Input: part model. Units: mm. Frame: model coordinates. A direction names the side the tool comes from. Round coordinates to 2 decimals unless told otherwise and drop trailing zeros. Write each loop counter-clockwise with the first axis right and the second up, starting at its lowest first coordinate (ties: lowest second). Pieces come first, ordered by that corner, then holes. Notation, with made-up numbers: (89, 72) - (125, 72) arc R25 cw to (125, 101) - close; hole circle Ø5 at (2, 3.25). An arc over 180 degrees is marked (long way). Use one line per item in the form item = value.
```python
from build123d import *

# Parameters (mm, degrees)
BOSS_EXTRUDE1_DEPTH  = 6.35
M5_CLEARANCE_HOLE1_D = 5.5
CUT_EXTRUDE2_DEPTH   = 7.35
FILLET1_R            = 10
M3_CLEARANCE_HOLE1_D = 3.4
SKETCH10_R           = 11.5
CUT_EXTRUDE3_DEPTH   = 7.35
FILLET2_R            = 5


with BuildPart() as part:
    # Sketch1 → Boss-Extrude1 (new body)
    with BuildSketch(Plane(origin=(0, 0, 0), x_dir=(1, 0, 0), z_dir=(0, 1, 0))):
        with BuildLine():
            Line((25.4, -25.4), (-25.4, -25.4))
            Line((-25.4, -25.4), (-25.4, 25.4))
            Line((-25.4, 25.4), (-25.4, 43.35))
            Line((-25.4, 43.35), (1.2, 43.35))
            Line((1.2, 43.35), (1.2, 25.4))
            Line((1.2, 25.4), (25.4, 25.4))
            Line((25.4, 25.4), (89.621209859, 25.4))
            Line((89.621209859, 25.4), (89.621209859, -50.04))
            Line((89.621209859, -50.04), (51.541941751, -50.04))
            ThreePointArc((51.541941751, -50.04), (44.870841587, -48.474895705), (39.591870426, -44.10618968))
            Line((39.591870426, -44.10618968), (25.4, -25.4))
        make_face()
    extrude(amount=BOSS_EXTRUDE1_DEPTH)

    # M5 Clearance Hole1 (through all)
    with Locations(Plane(origin=(0, 6.35, 0), x_dir=(1, 0, 0), z_dir=(0, 1, 0))):
        with Locations((-12.7, 12.7), (12.7, 12.7), (12.7, -12.7), (-12.7, -12.7), (-11.5, 38.1)):
            Hole(M5_CLEARANCE_HOLE1_D / 2)

    # Sketch7 → Cut-Extrude2 (cut, through all)
    with BuildSketch(Plane(origin=(0, 6.35, 0), x_dir=(1, 0, 0), z_dir=(0, 1, 0))):
        with BuildLine():
            Line((53.051764766, -31.105892862), (50.215452987, -32.745892862))
            ThreePointArc((50.215452987, -32.745892862), (49.247834614, -36.366488764), (52.868430515, -37.334107138))
            Line((52.868430515, -37.334107138), (55.704742294, -35.694107138))
            ThreePointArc((55.704742294, -35.694107138), (56.672360668, -32.073511236), (53.051764766, -31.105892862))
        make_face()
        with BuildLine():
            Line((33.75, -19.08), (33.75, -20.72))
            ThreePointArc((33.75, -20.72), (36.4, -23.37), (39.05, -20.72))
            Line((39.05, -20.72), (39.05, -19.08))
            ThreePointArc((39.05, -19.08), (36.4, -16.43), (33.75, -19.08))
        make_face()
    extrude(amount=-CUT_EXTRUDE2_DEPTH, mode=Mode.SUBTRACT)

    # Fillet1
    fillet1_edges = [part.edges().sort_by_distance(p)[0] for p in [
        (-25.4, 3.175, -43.35),
        (1.2, 3.175, -43.35),
        (89.621209859, 3.175, -25.4),
        (89.621209859, 3.175, 50.04),
        (25.4, 3.175, 25.4),
        (-25.4, 3.175, 25.4),
    ]]
    fillet(fillet1_edges, radius=FILLET1_R)

    # M3 Clearance Hole1 (through all)
    with Locations(Plane(origin=(0, 6.35, 0), x_dir=(1, 0, 0), z_dir=(0, 1, 0))):
        with Locations((50.121209859, 9.14), (81.121209859, 9.14), (81.121209859, -21.86), (50.121209859, -21.86)):
            Hole(M3_CLEARANCE_HOLE1_D / 2)

    # Sketch10 → Cut-Extrude3 (cut, through all)
    with BuildSketch(Plane(origin=(0, 6.35, 0), x_dir=(1, 0, 0), z_dir=(0, 1, 0))):
        with Locations((65.621209859, -6.36)):
            Circle(SKETCH10_R)
    extrude(amount=-CUT_EXTRUDE3_DEPTH, mode=Mode.SUBTRACT)

    # Fillet2
    fillet2_edges = [part.edges().sort_by_distance(p)[0] for p in [
        (1.2, 3.175, -25.4),
    ]]
    fillet(fillet2_edges, radius=FILLET2_R)


solid = part.part
```
(1) Cut plane A-A on y = 1.75. Count the separate pieces of the cut face and the enclosed holes in it, then the cut area to 3 significant figures.
Derived:
separate_pieces = 1
enclosed_holes = 12
area = 6,930 mm^2
(2) Material intervals for L1, parallel to X at y = 4, z = -9.14; L2, parallel to Z at x = 13, y = 0.75; L3, parallel to X at y = 1.5, z = -12.7, sorted ascending.
Derived:
L1 = -25.4 to 48.42, 51.82 to 79.42, 82.82 to 89.62
L2 = -25.4 to -15.43, -9.97 to 9.97, 15.43 to 25.4
L3 = -25.4 to -15.45, -9.95 to 9.95, 15.45 to 89.62
(3) Cut plane C-C on z = 12.7. Output: boundary loops of the cut face in (x, y).
Derived:
outline = (-25.4, 0) - (-15.45, 0) - (-15.45, 6.35) - (-25.4, 6.35) - close; (-9.95, 0) - (9.95, 0) - (9.95, 6.35) - (-9.95, 6.35) - close; (15.45, 0) - (56.03, 0) - (56.03, 6.35) - (15.45, 6.35) - close; (75.22, 0) - (89.62, 0) - (89.62, 6.35) - (75.22, 6.35) - close
(4) First-contact query: pin 1 Ø5 at (x, z) = (12.7, 12.7) entering from -Y; pin 2 Ø2.5 at (y, z) = (3.5, -32) entering from +X; pin 3 Ø0.5 at (y, z) = (3.5, 20) entering from -X; pin 4 Ø1.9 at (x, y) = (-5.5, 1.5) entering from +Z. Flat tips, straight axial feed; report the tip coordinate or a pass-through.
Derived:
pin_1 = through
pin_2 = 1.2
pin_3 = -24.4
pin_4 = 25.4
(5) Cut plane B-B on x = 12.7. Output: boundary loops of the cut face in (y, z), then the cut area to 3 significant figures.
Derived:
outline = (0, -25.4) - (6.35, -25.4) - (6.35, -15.45) - (0, -15.45) - close; (0, -9.95) - (6.35, -9.95) - (6.35, 9.95) - (0, 9.95) - close; (0, 15.45) - (6.35, 15.45) - (6.35, 25.4) - (0, 25.4) - close
area = 253 mm^2
(6) Cut plane D-D on x = 73.5. Output: boundary loops of the cut face in (y, z).
Derived:
outline = (0, -25.4) - (6.35, -25.4) - (6.35, -2.02) - (0, -2.02) - close; (0, 14.74) - (6.35, 14.74) - (6.35, 50.04) - (0, 50.04) - close
(7) Access query for faces 1 (the face through (33, 0, 3)), 2 (the face through (42, 3, -25.4)), 3 (the face through (36.46, 3.22, 16.43)). Directions: +Z, -Z, +X, -X, +Y, -Y. A direction counts if a zero-diameter tool reaches every point of the face in a straight line with its end or side. Return the directions, or none.
Derived:
face_1 = +Z, -Z, +X, -X, -Y
face_2 = -Z, +X, +Y, -Y
face_3 = +Y, -Y
(8) Draft query along X for faces 4 (the face through (89.621, 3, 12)), 5 (the face through (44.96, 3.13, 48.52)), 6 (the face through (-12.104, 3.131, 15.385)). Return one class per face: released by +X, released by -X, zero draft, split by the parting line, or undercut.
Derived:
face_4 = released by +X
face_5 = released by -X
face_6 = undercut
